Autodesk Inventor part; units mm, degrees
ref_plane "YZ Plane" through (0, 0, 0) normal (1, 0, 0) x (0, 1, 0)
ref_plane "XZ Plane" through (0, 0, 0) normal (0, 1, 0) x (-1, 0, 0)
ref_plane "XY Plane" through (0, 0, 0) normal (0, 0, 1) x (1, 0, 0)
sketch "스케치1" plane through (0, 0, 0) normal (0, 0, 1) x (1, 0, 0)
  circle A0 centre (0, 0) radius 80
  circle A1 centre (0, 0) radius 34 construction
  circle A2 centre (0, 0) radius 27
  circle A3 centre (0, 0) radius 60
  circle A4 centre (0, 0) radius 40
  line L0 (0, 0) -> (22.961, 55.4328)
  line L1 (0, 0) -> (55.4328, 22.961)
  line L2 (0, 0) -> (0, 60) construction
  point P0 (15.3073, 36.9552)
  point P1 (36.9552, 15.3073)
  dimension "d0" = 160
  dimension "d1" = 68
  dimension "d2" = 54
  dimension "d3" = 120
  dimension "d4" = 80
  dimension "d5" = 45
  dimension "d45" = 22.5
extrude "돌출1" add sketch "스케치1" along normal blind 5 contours A0 | A2 L1 A4 L0 | A2 L0 A4 L1 | L1 A3 L0 A4 | A4 L0 A3 L1
extrude "돌출2" cut sketch "스케치1" along normal blind 5 contours A4 L0 A3 L1 picked at (23.2061, 47.8488)
fillet "모깎기1" radius 4 4 edges at (22.961, 55.4328, 2.5) (15.3073, 36.9552, 2.5) (36.9552, 15.3073, 2.5) (55.4328, 22.961, 2.5)
sketch "스케치2" plane through (0, 0, 5) normal (0, 0, 1) x (1, 0, 0)
  circle A0 centre (0, 70) radius 1.75
  point P0 (0, 0)
  dimension "d14" = 3.5
  dimension "d15" = 70
extrude "돌출3" cut sketch "스케치2" against normal blind 5
pattern_circular "원형 패턴2" count 4 over 360 about axis through (0, 0, 0) along (0, 0, 1) of "돌출3"
sketch "스케치3" plane through (0, 0, 5) normal (0, 0, 1) x (1, 0, 0)
  circle A0 centre (0, 0) radius 6 construction
  line L0 (-6, 16.5) -> (6, 16.5) construction
  line L1 (6, 16.5) -> (6, -6) construction
  line L2 (6, -6) -> (-6, -6) construction
  line L3 (-6, -6) -> (-6, 16.5) construction
  line L4 (-6, 21.35) -> (6, 21.35) construction
  line L5 (6, 21.35) -> (6, -10.85) construction
  line L6 (6, -10.85) -> (-6, -10.85) construction
  line L7 (-6, -10.85) -> (-6, 21.35) construction
  circle A1 centre (0, 19.35) radius 0.75
  line L8 (-6, 5.25) -> (-8.8851, 5.25) construction
  circle A2 centre (0, -8.85) radius 0.75
  line L9 (-6, 27) -> (6, 27)
  line L10 (6, 27) -> (6, 17)
  line L11 (6, 17) -> (-6, 17)
  line L12 (-6, 17) -> (-6, 27)
  line L13 (-6, -6.5) -> (6, -6.5)
  line L14 (6, -6.5) -> (6, -27)
  line L15 (6, -27) -> (-6, -27)
  line L16 (-6, -27) -> (-6, -6.5)
  circle A3 centre (0, 0) radius 27
  point P0 (0, -6)
  point P1 (0, 27)
  point P2 (0, -27)
  point P3 (-6, -26.3249)
  point P4 (6, -26.3249)
  point P5 (6, 26.3249)
  point P6 (-6, 26.3249)
  dimension "d21" = 12
  dimension "d22" = 12
  dimension "d23" = 22.5
  dimension "d24" = 32.2
  dimension "d26" = 1.5
  dimension "d27" = 28.2
  dimension "d28" = 0.5
  dimension "d29" = 0.5
  dimension "d30" = 12
  dimension "d31" = 12
extrude "돌출4" add sketch "스케치3" against normal blind 5 contours A3 L10 L11 L12 | L16 L13 L14 A3
fillet "모깎기2" radius 4 4 edges at (-6, 26.3249, 2.5) (6, 26.3249, 2.5) (-6, -26.3249, 2.5) (6, -26.3249, 2.5)
sketch "스케치4" plane through (0, 0, 0) normal (0, 0, -1) x (-1, 0, 0)
  circle A0 centre (0, 0) radius 32.0565 construction
  circle A1 centre (0, -32.0565) radius 0.75
  line L0 (0, -32.0565) -> (0, 0)
  line L1 (0, 0) -> (29.6163, -12.2675)
  circle A2 centre (29.6163, -12.2675) radius 0.75
  circle A3 centre (0, 32.0565) radius 0.75
  circle A4 centre (-29.6163, 12.2675) radius 0.75
  dimension "d35" = 64.113
  dimension "d36" = 1.5
  dimension "d37" = 1.5
  dimension "d38" = 67.5
  dimension "d41" = 360
extrude "돌출5" cut sketch "스케치4" against normal blind 5
mirror "미러1" about plane through (0, 0, 0) normal (1, 0, 0) of "돌출2", "모깎기1"
properties part number "아크릴 LED확산판"
Here's how the part is built. I have some questions about the finished solid (model axes, mm). A direction names the side the tool comes from. Give positions to 0.01 mm unless a question says otherwise; leave off trailing zeros. Order: outer loops, then holes, each group sorted by start corner. A loop starts at its lowest first (then second) coordinate and runs counter-clockwise, first axis right, second up. Notation, with made-up numbers: (-24, 22.5) -> (28, 22.5) arc R33 cw to (28, 51.5) -> close; hole circle Ø6 at (74.5, 48.25). An arc over 180 degrees is marked (long way). One line per item, written item: value. Start each with the question number.
1. Imagine slicing it at C-C, the plane y = -35.5. List the corners of the cut face in (x, z) for me, plus the area to 3 significant figures.
2. For faces 1 (the face through (28.165, 28.403, 2.465)), 2 (the face through (-1, -17, 5)), which set-ups out of +Z, -Z, +X, -X, +Y, -Y let a thin tool reach every point of the face, with its end or its side?
3. Will these pins go through, and if not, where does the flat tip stop? pin 1 Ø1.1 at (y, z) = (19, 3) entering from -X; pin 2 Ø1.5 at (y, z) = (-11, 3.5) entering from +X; pin 3 Ø2.5 at (x, z) = (1, 3.5) entering from +Y; pin 4 Ø3 at (x, y) = (0, 70) entering from -Z.
4. Imagine slicing it at A-A, the plane x = -42.5. List the corners of the cut face in (y, z) for me.
5. We'd pull the mould along X, two halves only. Please class faces 3 (the face through (45.97, 19.04, 2.46)), 4 (the face through (-17.34, 78.1, 2.46)), 5 (the face through (-1, -17, 0)): released by +X, released by -X, zero draft, split by the parting line, or undercut.
6. Imagine slicing it at B-B, the plane z = 1.45. Count the separate pieces of the cut face and the enclosed holes in it, plus the area to 3 significant figures.
7. I need wall thicknesses on probe 1 along X at (y, z) = (38, 1.5); probe 2 along Y at (x, z) = (22.5, 0.7); probe 3 along Y at (x, z) = (14.5, 2.05). Which ranges of each line are inside material? Lowest first, please. Write a range as from..to.
Values follow:
1. outline: (-71.69, 0) -> (71.69, 0) -> (71.69, 5) -> (-71.69, 5) -> close
1. area: 717 mm2
2. face 1: +Z, -Z
2. face 2: +Z, +X, -X, +Y, -Y
3. pin 1: stops at x = -77.84
3. pin 2: stops at x = 79.34
3. pin 3: stops at y = 80
3. pin 4: passes through
4. outline: (-67.78, 0) -> (17.6, 0) -> (17.6, 5) -> (-67.78, 5) -> close; (42.35, 0) -> (67.78, 0) -> (67.78, 5) -> (42.35, 5) -> close
5. face 3: undercut
5. face 4: split by the parting line
5. face 5: zero draft
6. separate pieces: 1
6. enclosed holes: 13
6. area: 16,600 mm2
7. probe 1: x = -70.4..-46.43, -16.58..16.58, 46.43..70.4
7. probe 2: y = -76.77..-14.92, 14.92..33.07, 53.14..76.77
7. probe 3: y = -78.67..-22.78, 22.78..78.67
